Build history of the part. All positions in model axes, mm. Give positions to 0.01 mm unless a question says otherwise; leave off trailing zeros. Write each loop counter-clockwise with the first axis right and the second up, starting at its lowest first coordinate (ties: lowest second). Pieces come first, ordered by that corner, then holes. Notation, with made-up numbers: (-3.75, 79) -> (52.25, 79) arc R15 cw to (52.25, 108) -> close; hole circle Ø1 at (32, 5). An arc over 180 degrees is marked (long way). Put each result on its own line as item: value. Start each with the question number.
Item 1: Drill centre lines: line 1 along Z through (x, y) = (-1168, -95); line 2 along Y through (x, z) = (-1159.5, 10.5); line 3 along Z through (x, y) = (-1169, -71). Where is each one in solid material? Low to high.
Item 2: Slice it at A-A, the plane y = -95.25. List the corners of the cut face in (x, z).
Item 3: Slice it at C-C, the plane x = -1178. List the corners of the cut face in (y, z) (3 decimals), plus the area to 3 significant figures.
Item 4: Flat gauge pin, fed straight in: pin 1 Ø15 at (y, z) = (-95.25, -10.46) entering from +X. Where does the tip first touch, or does it go through?
Item 5: Slice it at B-B, the plane z = -6.5. List the corners of the cut face in (x, y), plus the area to 3 significant figures.
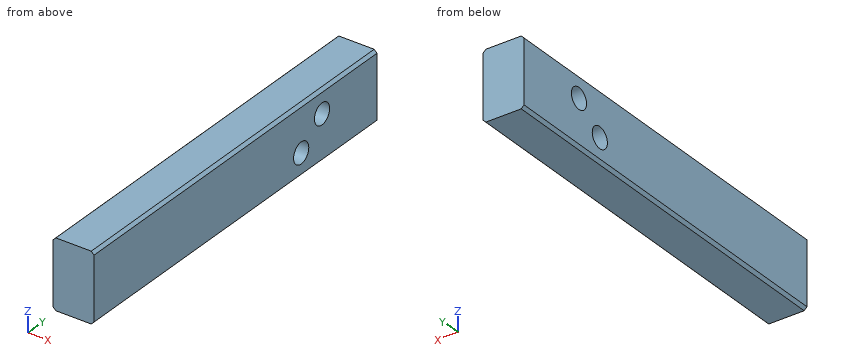
```python
from build123d import *

# Parameters (mm, degrees)
F0_W     = 37.30498
F0_H     = 62.70498
F1_DEPTH = 355.6
F3_D     = 19.05
F4_SIZE  = 2.54


with BuildPart() as f1:
    # F0 (on Front) → F1 (new body)
    with BuildSketch(Plane.XZ):
        with Locations((-1175.14751, 0)):
            Rectangle(F0_W, F0_H)
    extrude(amount=F1_DEPTH)

    # F3 (through all)
    with Locations(Plane(origin=(-1193.8, 0, 0), x_dir=(0, -1, 0), z_dir=(-1, 0, 0))):
        with Locations((69.05498, 10.44829), (95.25, -10.45591)):
            Hole(F3_D / 2)

    # F4
    f4_edges = [f1.edges().sort_by_distance(p)[0] for p in [
        (-1193.8, -177.8, 31.35249),
        (-1156.49502, -177.8, 31.35249),
        (-1193.8, -177.8, -31.35249),
        (-1156.49502, -177.8, -31.35249),
    ]]
    chamfer(f4_edges, length=F4_SIZE)


solid = f1.part
```
Values follow:
1. line 1: -31.35 to -19.98, -0.93 to 31.35
1. line 2: -355.6 to -78.58, -59.53 to 0
1. line 3: -31.35 to 1.12, 19.77 to 31.35
2. outline: (-1193.8, -28.81) -> (-1191.26, -31.35) -> (-1159.04, -31.35) -> (-1156.5, -28.81) -> (-1156.5, -19.98) -> (-1193.8, -19.98) -> close; (-1193.8, -0.93) -> (-1156.5, -0.93) -> (-1156.5, 28.81) -> (-1159.04, 31.35) -> (-1191.26, 31.35) -> (-1193.8, 28.81) -> close
3. outline: (-355.6, -31.352) -> (0, -31.352) -> (0, 31.352) -> (-355.6, 31.352) -> close; hole circle Ø19.05 at (-95.25, -10.456); hole circle Ø19.05 at (-69.055, 10.448)
3. area: 21,700 mm2
4. pin 1: through
5. outline: (-1193.8, -355.6) -> (-1156.5, -355.6) -> (-1156.5, -103.91) -> (-1193.8, -103.91) -> close; (-1193.8, -86.59) -> (-1156.5, -86.59) -> (-1156.5, 0) -> (-1193.8, 0) -> close
5. area: 12,600 mm2
